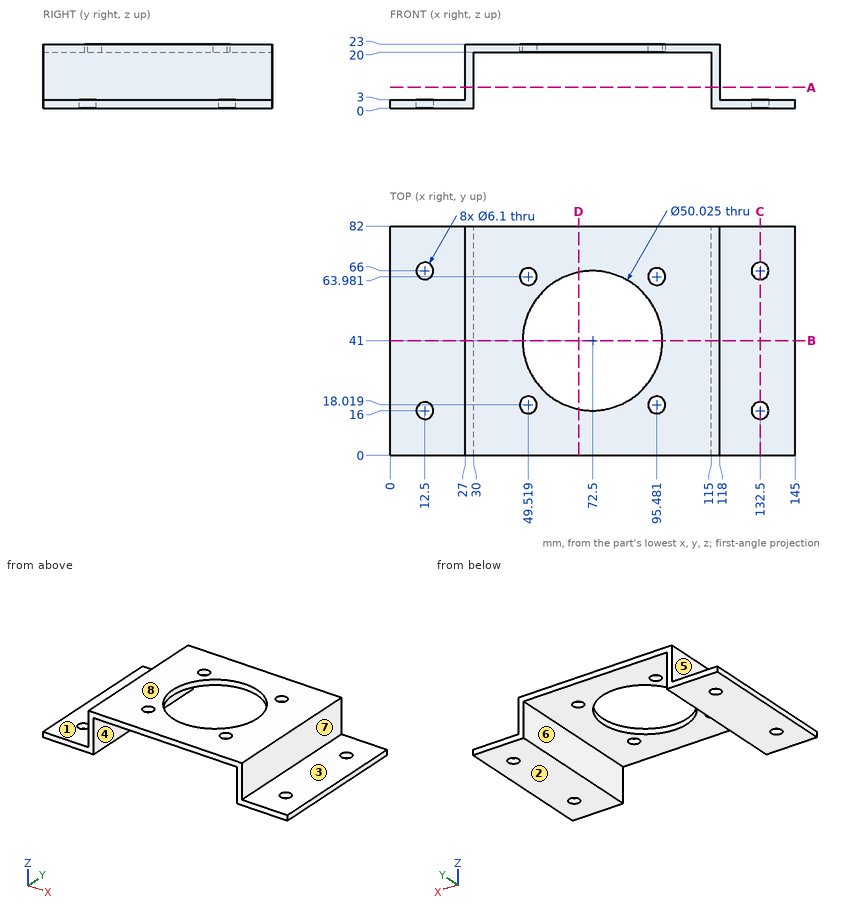
Answer from the drawing. Dimensions are ordinates in mm from the lowest x, y and z of the part. A direction names the side the tool comes from. Coordinates: 2 decimals unless noted, no trailing zeros. Order: outer loops, then holes, each group sorted by start corner. A loop starts at its lowest first (then second) coordinate and runs counter-clockwise, first axis right, second up. Notation, with made-up numbers: (-35.75, 52.25) -> (-16.75, 52.25) arc R14 cw to (-16.75, 63.25) -> close; hole circle Ø10 at (5, 79). An arc over 180 degrees is marked (long way). Answer as a JSON object with one key per item and string values.
1) A cutting plane is placed at B-B, the plane y = 41. Determine the outline of the cut face in (x, z).
Model answer:
{"outline": "(0, 0) -> (30, 0) -> (30, 20) -> (47.49, 20) -> (47.49, 23) -> (27, 23) -> (27, 3) -> (0, 3) -> close; (97.51, 20) -> (115, 20) -> (115, 0) -> (145, 0) -> (145, 3) -> (118, 3) -> (118, 23) -> (97.51, 23) -> close"}
2) A cutting plane is placed at D-D, the plane x = 67.5. Determine the outline of the cut face in (y, z), plus the area to 3 significant figures.
Model answer:
{"outline": "(0, 20) -> (16.49, 20) -> (16.49, 23) -> (0, 23) -> close; (65.51, 20) -> (82, 20) -> (82, 23) -> (65.51, 23) -> close", "area": "99.0 mm²"}
3) A tool of negligible diameter and unlimited length cuts with its end or side. For the marked faces 1, 2, 3 and 4, from which of +Z, -Z, +X, -X, +Y, -Y can it reach the whole face along a straight path? Write none if from no direction.
Model answer:
{"face 1": "+Z, -X, +Y, -Y", "face 2": "-Z, +X, -X, +Y, -Y", "face 3": "+Z, +X, +Y, -Y", "face 4": "-Z, +Y, -Y"}
4) Consider line 1 along Y through (x, z) = (132.5, 1.7); line 2 along X through (y, z) = (46.5, 7.5); line 3 along X through (y, z) = (77, 1.25). Determine where each line is inside the solid, lowest interval first. Write a range as from..to.
Model answer:
{"line 1": "y = 0..12.95, 19.05..62.95, 69.05..82", "line 2": "x = 27..30, 115..118", "line 3": "x = 0..30, 115..145"}
5) A cutting plane is placed at A-A, the plane z = 7.5. Determine the outline of the cut face in (x, y), plus the area to 3 significant figures.
Model answer:
{"outline": "(27, 0) -> (30, 0) -> (30, 82) -> (27, 82) -> close; (115, 0) -> (118, 0) -> (118, 82) -> (115, 82) -> close", "area": "492 mm²"}
6) Each of these flat-tipped pins is pushed along its axis until it touches: pin 1 (6 mm diameter, centred on x = 111.5, y = 20, fed in from -Z); pin 2 (10 mm diameter, centred on y = 46, z = 12.5, fed in from -X); pin 3 (21.5 mm diameter, centred on x = 136.5, y = 29.5, fed in from +Z). Where does it stop, or does it pass through?
Model answer:
{"pin 1": "stops at z = 20", "pin 2": "stops at x = 27", "pin 3": "stops at z = 3"}
7) A cutting plane is placed at C-C, the plane x = 132.5. Determine the outline of the cut face in (y, z).
Model answer:
{"outline": "(0, 0) -> (12.95, 0) -> (12.95, 3) -> (0, 3) -> close; (19.05, 0) -> (62.95, 0) -> (62.95, 3) -> (19.05, 3) -> close; (69.05, 0) -> (82, 0) -> (82, 3) -> (69.05, 3) -> close"}
8) The mould has two halves that part along X. Classify the marked faces 5, 6, 7 and 8: released by +X, released by -X, zero draft, split by the parting line, or undercut.
Model answer:
{"face 5": "released by -X", "face 6": "undercut", "face 7": "released by +X", "face 8": "zero draft"}
